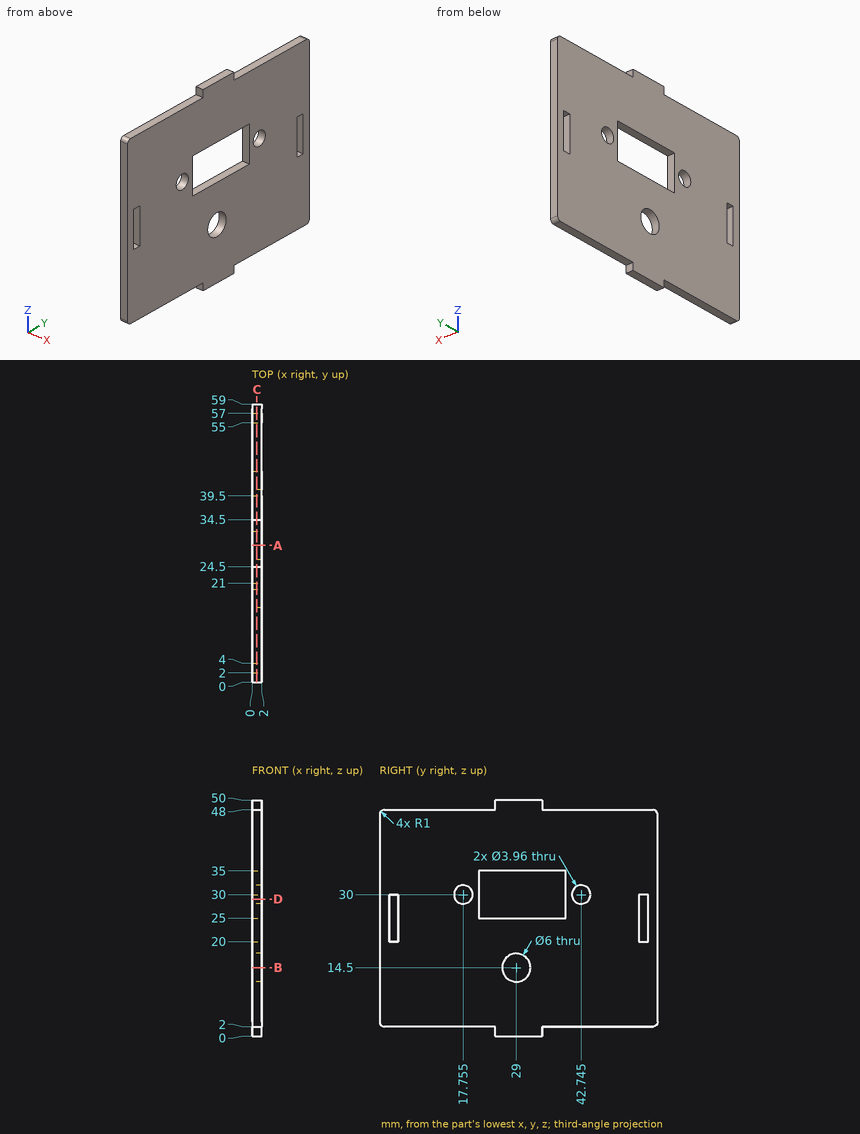
The figure shows three views and two pictorial views of one solid part (mm, origin at its lowest corner). Answer the questions. Give positions to 0.01 mm unless a question says otherwise; leave off trailing zeros. Write each loop counter-clockwise with the first axis right and the second up, starting at its lowest first coordinate (ties: lowest second). Pieces come first, ordered by that corner, then holes. Notation, with made-up numbers: M -11.5,40.5 L -2.5,40.5 A8 ccw -2.5,54.5 Z; hole C -18,58 d3. An arc over 180 degrees is marked long. Write each question's results on one line, items separated by ' | '.
Q1. Flat-ended cylindrical pins translate along their axes: P1, Ø0.6, axis at x = 1, z = 49, coming from the +Y side; P2, Ø0.6, axis at x = 1.5, z = 1, coming from the -Y side; P3, Ø1, axis at x = 1, y = 47.5, coming from the +Z side. Find the tip coordinate at first contact, or state that the pin passes through.
Output values:
P1: y = 34.5 | P2: y = 24.5 | P3: z = 48
Q2. Section B-B, the plane z = 14.5 is taken. Write down the section's boundary in (x, y), then the cut area to 3 significant figures.
Output values:
outline: M 0,0 L 2,0 L 2,26 L 0,26 Z; M 0,32 L 2,32 L 2,59 L 0,59 Z | area: 106 mm2
Q3. Consider L1, parallel to Z at x = 1.4, y = 29; L2, parallel to Y at x = 1.9, z = 32.5; L3, parallel to Z at x = 1.7, y = 38. Determine where each line is inside the solid, lowest interval first. Write a range as from..to.
Output values:
L1: 0..11.5, 17.5..25, 35..50 | L2: 0..21, 39.5..59 | L3: 2..25, 35..48
Q4. Section C-C, the plane x = 1 is taken. Count the separate pieces of the cut face and the enclosed holes in it, then the cut area to 3 significant figures.
Output values:
separate pieces: 1 | enclosed holes: 6 | area: 2,480 mm2
Q5. Section A-A, the plane y = 29 is taken. Write down the section's boundary in (x, z).
Output values:
outline: M 0,0 L 2,0 L 2,11.5 L 0,11.5 Z; M 0,17.5 L 2,17.5 L 2,25 L 0,25 Z; M 0,35 L 2,35 L 2,50 L 0,50 Z
Q6. Section D-D, the plane z = 29 is taken. Write down the section's boundary in (x, y), then the cut area to 3 significant figures.
Output values:
outline: M 0,0 L 2,0 L 2,2 L 0,2 Z; M 0,4 L 2,4 L 2,16.05 L 0,16.05 Z; M 0,19.46 L 2,19.46 L 2,21 L 0,21 Z; M 0,39.5 L 2,39.5 L 2,41.04 L 0,41.04 Z; M 0,44.45 L 2,44.45 L 2,55 L 0,55 Z; M 0,57 L 2,57 L 2,59 L 0,59 Z | area: 59.3 mm2
